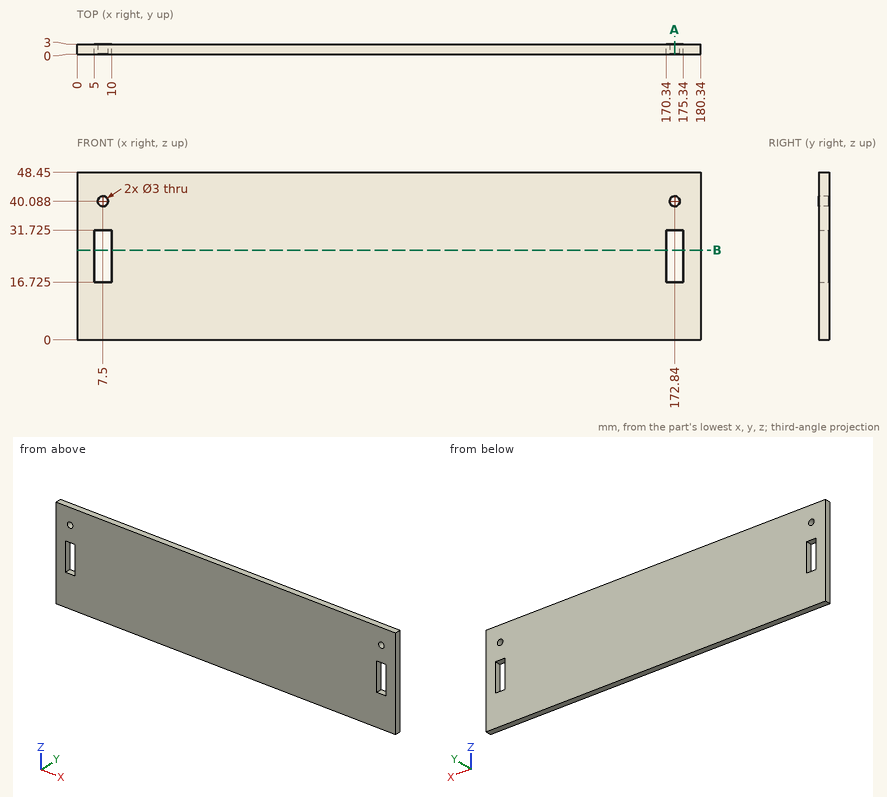
Design review of the part shown in the three views and the two pictorial views. Dimensions are in mm from the part's minimum x, y and z. Round coordinates to 2 decimals unless told otherwise and drop trailing zeros. Loops run counter-clockwise (first coordinate to the right, second up) from the corner with the lowest first, then second, coordinate; pieces in that order, holes last. Notation, with made-up numbers: (39.5, 59.25) -> (95.5, 59.25) arc R30 ccw to (95.5, 83.25) -> close; hole circle Ø7 at (49.5, -8). An arc over 180 degrees is marked (long way). Answer as CSV lines item,"result".
1) Add section B-B on z = 26. Write out the cut boundary in (x, y), plus the area to 3 significant figures.
Geometry results:
outline,"(0, 0) -> (5, 0) -> (5, 3) -> (0, 3) -> close; (10, 0) -> (170.34, 0) -> (170.34, 3) -> (10, 3) -> close; (175.34, 0) -> (180.34, 0) -> (180.34, 3) -> (175.34, 3) -> close"
area,"511 mm²"
2) Add section A-A on x = 172.84. State how many separate pieces and enclosed holes the cut face has.
Geometry results:
separate pieces,"3"
enclosed holes,"0"
3) To check wall thickness, follow line 1 along X through (y, z) = (1.35, 19); line 2 along X through (y, z) = (0.35, 40). State the ranges of each line that lie inside material, in increasing order. Write a range as from..to.
Geometry results:
line 1,"x = 0..5, 10..170.34, 175.34..180.34"
line 2,"x = 0..6, 9..171.34, 174.34..180.34"
4) For P1, Ø1, axis at x = 25.5, z = 14, coming from the -Y side; P2, Ø2.5, axis at x = 172.84, z = 40.09, coming from the +Y side, all flat-tipped, find the tip position at first contact; note any pin that passes through.
Geometry results:
P1,"stops at y = 0"
P2,"passes through"
